Answer from the drawing. Dimensions are ordinates in mm from the lowest x, y and z of the part. A direction names the side the tool comes from. Coordinates: 2 decimals unless noted, no trailing zeros. Loops run counter-clockwise (first coordinate to the right, second up) from the corner with the lowest first, then second, coordinate; pieces in that order, holes last. Notation, with made-up numbers: (89.25, -29.75) -> (146.25, -29.75) arc R13 ccw to (146.25, -15.75) -> close; hole circle Ø5 at (15.25, -26.5). An arc over 180 degrees is marked (long way). Use a Markdown table: item, result.
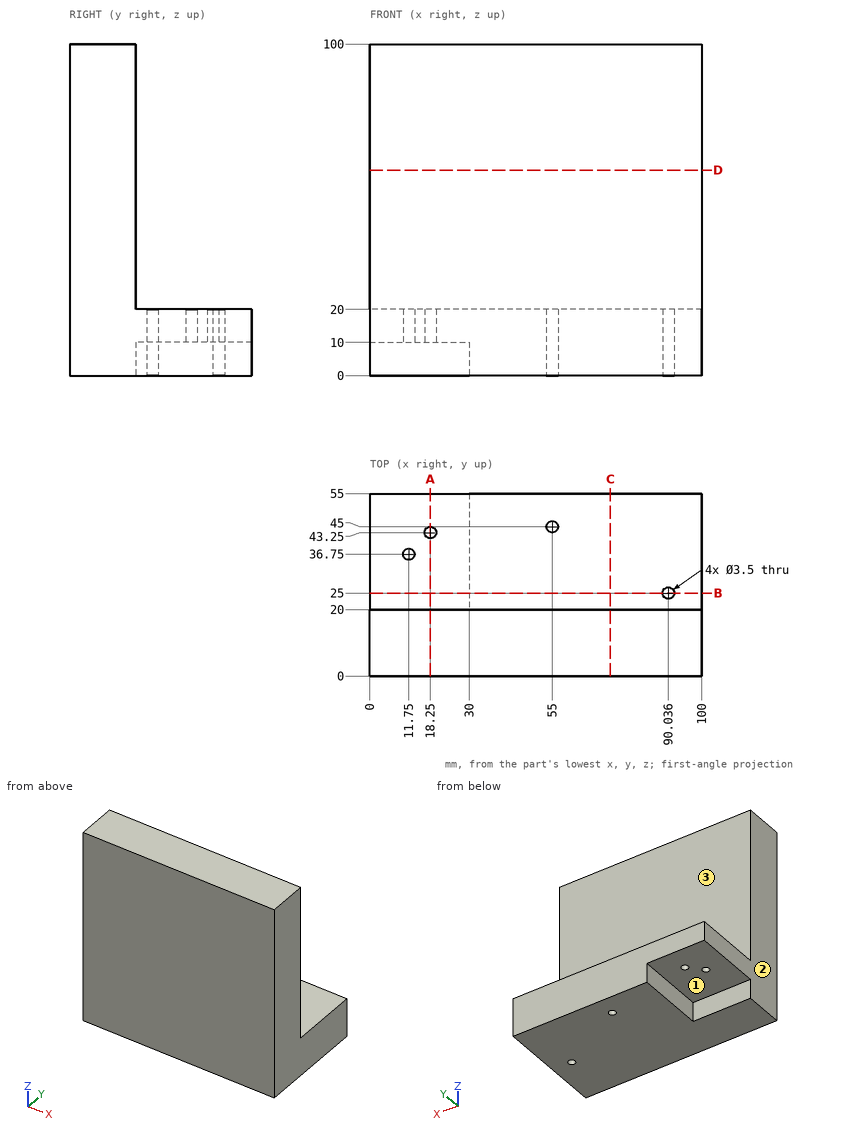
Q1. Section D-D on z = 62 is taken. Determine the outline of the cut face in (x, y), and give its area (3 significant figures).
Solved:
| item | result |
|---|---|
| outline | (0, 0) -> (100, 0) -> (100, 20) -> (0, 20) -> close |
| area | 2,000 mm² |
Q2. Given pin 1 Ø11 at (x, z) = (20.5, 4) entering from +Y; pin 2 Ø9 at (x, y) = (19.5, 45.5) entering from -Z; pin 3 Ø10 at (x, z) = (73, 35.5) entering from -Y; pin 4 Ø5.5 at (x, y) = (55, 45) entering from +Z, each flat-ended and moving along its own axis, determine where each tip first touches the part or whether it passes through.
Solved:
| item | result |
|---|---|
| pin 1 | y = 20 |
| pin 2 | z = 10 |
| pin 3 | y = 0 |
| pin 4 | z = 20 |
Q3. Section A-A on x = 18.25 is taken. Determine the outline of the cut face in (y, z).
Solved:
| item | result |
|---|---|
| outline | (0, 0) -> (20, 0) -> (20, 10) -> (41.5, 10) -> (41.5, 20) -> (20, 20) -> (20, 100) -> (0, 100) -> close; (45, 10) -> (55, 10) -> (55, 20) -> (45, 20) -> close |
Q4. Consider line 1 (X direction, y = 25, z = 13); line 2 (X direction, y = 43, z = 15); line 3 (Y direction, x = 11.75, z = 15). Determine where each line is inside the solid, lowest interval first. Write a range as [from, to].
Solved:
| item | result |
|---|---|
| line 1 | [0, 88.29], [91.79, 100] |
| line 2 | [0, 16.52], [19.98, 100] |
| line 3 | [0, 35], [38.5, 55] |
Q5. Section C-C on x = 72.5 is taken. Determine the outline of the cut face in (y, z).
Solved:
| item | result |
|---|---|
| outline | (0, 0) -> (55, 0) -> (55, 20) -> (20, 20) -> (20, 100) -> (0, 100) -> close |
Q6. For the marked faces 1, 2 and 3, determine the directions among +Z, -Z, +X, -X, +Y, -Y from which every point of the face is accessible in a straight line to the end or side of a thin tool.
Solved:
| item | result |
|---|---|
| face 1 | -Z, -X, +Y |
| face 2 | +Z, -Z, -X, +Y, -Y |
| face 3 | +Z, +X, -X, +Y |
Q7. Section B-B on y = 25 is taken. Determine the outline of the cut face in (x, z), and give its area (3 significant figures).
Solved:
| item | result |
|---|---|
| outline | (0, 10) -> (30, 10) -> (30, 0) -> (88.29, 0) -> (88.29, 20) -> (0, 20) -> close; (91.79, 0) -> (100, 0) -> (100, 20) -> (91.79, 20) -> close |
| area | 1,630 mm² |
